Verification items for this drawing (mm, ordinates from the low corner). Round coordinates to 2 decimals unless told otherwise and drop trailing zeros. Loops run counter-clockwise (first coordinate to the right, second up) from the corner with the lowest first, then second, coordinate; pieces in that order, holes last. Notation, with made-up numbers: (78.5, -37.5) - (121.5, -37.5) arc R28 ccw to (121.5, -3.5) - close; hole circle Ø4 at (76.25, 10.5). An arc over 180 degrees is marked (long way). Answer in a Markdown table with one row per item. Add a question column.
(1) Cross-section at B-B on y = 6.5. Enter the section's corners in (x, z), then the cut area to 3 significant figures.
(2) Thickness scan on line 1 along X through (y, z) = (3, 19); line 2 along Y through (x, z) = (13, 87). Record the ranges inside material, lowest first.
(3) Cross-section at A-A on x = 30. Enter the section's corners in (y, z).
(4) Cross-section at C-C on z = 50.5. Enter the section's corners in (x, y).
(5) Gauge pin test, flat end, axial feed: pin 1 (5 mm diameter, centred on x = 26, y = 3, fed in from -Z). Record the tip position at first contact, or that the pin passes through.
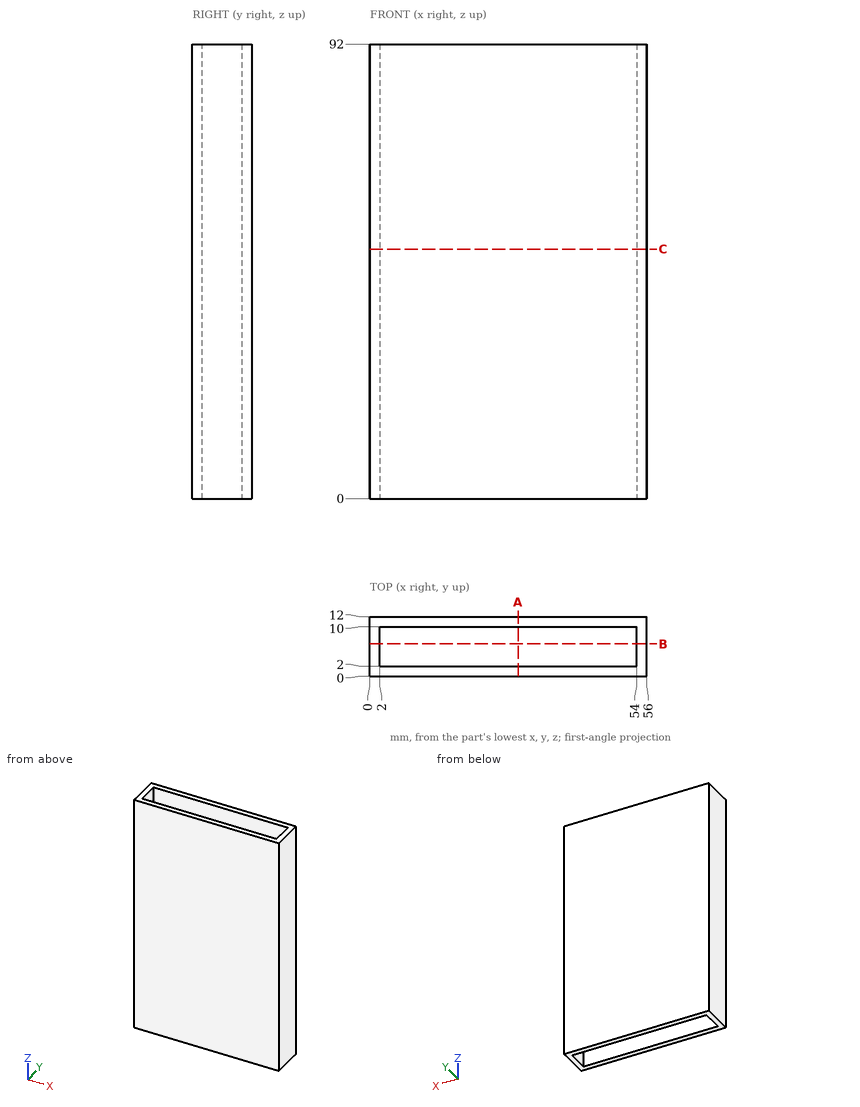
Answers:
| question | item | result |
|---|---|---|
| 1 | outline | (0, 0) - (2, 0) - (2, 92) - (0, 92) - close; (54, 0) - (56, 0) - (56, 92) - (54, 92) - close |
| 1 | area | 368 mm^2 |
| 2 | line 1 | x = 0 to 2, 54 to 56 |
| 2 | line 2 | y = 0 to 2, 10 to 12 |
| 3 | outline | (0, 0) - (2, 0) - (2, 92) - (0, 92) - close; (10, 0) - (12, 0) - (12, 92) - (10, 92) - close |
| 4 | outline | (0, 0) - (56, 0) - (56, 12) - (0, 12) - close; hole (2, 2) - (54, 2) - (54, 10) - (2, 10) - close |
| 5 | pin 1 | stops at z = 0 |
